```python
from build123d import *

# Parameters (mm, degrees)
F0_W     = 146.05
F0_H     = 41.91
F0_W_2   = 144.78
F0_H_2   = 40.64
F1_DEPTH = 184.15
F2_R     = 12.7
F3_DEPTH = 0.635
F4_W     = 25.654
F4_H     = 44.958
F4_W_2   = 14.224
F4_H_2   = 13.208
F4_R     = 10.16
F4_R_2   = 6.35
F4_R_3   = 2.54
F5_DEPTH = 0.635
F4_R_4   = 1.4859
F6_DEPTH = 0.635


with BuildPart() as f1:
    # F0 (on Front) → F1 (new body)
    with BuildSketch(Plane.XZ):
        with Locations((73.025, 20.955)):
            Rectangle(F0_W, F0_H)
        with Locations((73.025, 20.955)):
            Rectangle(F0_W_2, F0_H_2, mode=Mode.SUBTRACT)
    extrude(amount=-F1_DEPTH)

    # F2 (on face) → F3 (cut, through all)
    with BuildSketch(Plane(origin=(0, 0, 0), x_dir=(1, 0, 0), z_dir=(0, 0, -1))):
        with Locations((19.05, -165.1)):
            Circle(F2_R)
    extrude(amount=-F3_DEPTH, mode=Mode.SUBTRACT)

    # F4 (on face) → F5 (cut, through all)
    with BuildSketch(Plane.XY.offset(41.91)):
        with Locations((25.4, 48.9712)):
            Rectangle(F4_W, F4_H)
        with Locations((25.4, 103.4542)):
            Rectangle(F4_W_2, F4_H_2)
        with Locations((25.4, 148.59)):
            Circle(F4_R)
        with Locations((63.5, 92.075)):
            Circle(F4_R_2)
        with Locations((63.5, 57.785)):
            Circle(F4_R_3)
        with Locations((120.65, 71.755)):
            Circle(F4_R_3)
        with Locations((120.65, 132.715)):
            Circle(F4_R_3)
    extrude(amount=-F5_DEPTH, mode=Mode.SUBTRACT)

    # F4 (on face) → F6 (cut, through all)
    with BuildSketch(Plane.XY.offset(41.91)):
        with Locations((25.4, 130.5941)):
            Circle(F4_R_4)
        with Locations((63.5, 126.365)):
            Circle(F4_R_3)
        with Locations((120.65, 102.235)):
            Circle(F4_R_3)
        with Locations((120.65, 41.275)):
            Circle(F4_R_3)
    extrude(amount=-F6_DEPTH, mode=Mode.SUBTRACT)


solid = f1.part
```
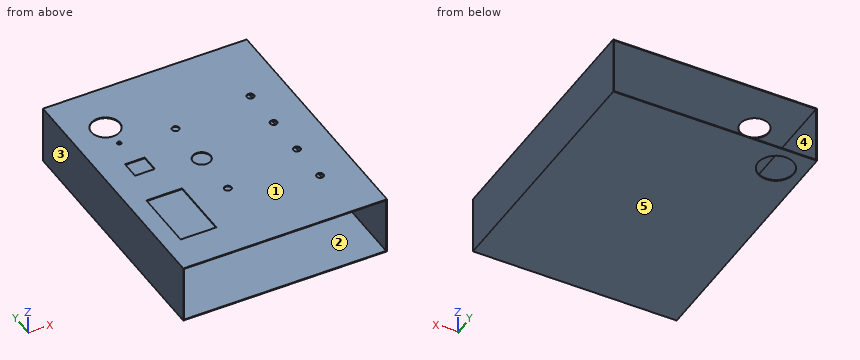
CAD build for the part. Positions are in the model's coordinates, mm. Face numbers are marked on the shaded views. A direction names the side the tool comes from. Round coordinates to 2 decimals unless told otherwise and drop trailing zeros. Order: outer loops, then holes, each group sorted by start corner. A loop starts at its lowest first (then second) coordinate and runs counter-clockwise, first axis right, second up. Notation, with made-up numbers: (43.5, 57.25) -> (62.5, 57.25) arc R26 ccw to (62.5, 79.25) -> close; hole circle Ø9 at (3, -5.5). An arc over 180 degrees is marked (long way). One line per question, with ' | ' between items.
Q1. Slice it at C-C (z = 22.5). Write the cut outline in (x, y) (3 decimals), then the cut area to 3 significant figures.
Completed:
outline: (0, 0) -> (0.635, 0) -> (0.635, 184.15) -> (0, 184.15) -> close; (145.415, 0) -> (146.05, 0) -> (146.05, 184.15) -> (145.415, 184.15) -> close | area: 234 mm^2
Q2. Two-plate mould, pull along Z, no slides. Class the marked faces 3, 4 and 5: released by +Z, released by -Z, zero draft, split by the parting line, or undercut.
Completed:
face 3: zero draft | face 4: undercut | face 5: released by -Z
Q3. Which spindle directions (+Z, -Z, +X, -X, +Y, -Y) get a long thin tool onto all of the face, cutting with end or side? Do the marked faces 1 and 2. Say none if no direction does.
Completed:
face 1: +Z, +X, -X, +Y, -Y | face 2: +Y, -Y
Q4. Slice it at B-B (y = 14). Write the cut outline in (x, z) (3 decimals), then the cut area to 3 significant figures.
Completed:
outline: (0, 0) -> (146.05, 0) -> (146.05, 41.91) -> (0, 41.91) -> close; hole (0.635, 0.635) -> (145.415, 0.635) -> (145.415, 41.275) -> (0.635, 41.275) -> close | area: 237 mm^2
Q5. Probe probe 1 along Y at (x, z) = (120.65, 41.4) (3 decimals); probe 2 along X at (y, z) = (83, 22) (3 decimals); probe 3 along Z at (x, y) = (114, 39.5) (3 decimals). List the from-to ranges inside material, lowest first.
Completed:
probe 1: y = 0 to 38.735, 43.815 to 69.215, 74.295 to 99.695, 104.775 to 130.175, 135.255 to 184.15 | probe 2: x = 0 to 0.635, 145.415 to 146.05 | probe 3: z = 0 to 0.635, 41.275 to 41.91
Q6. Slice it at D-D (y = 148.59). Write the cut outline in (x, z) (3 decimals), then the cut area to 3 significant figures.
Completed:
outline: (0, 0) -> (146.05, 0) -> (146.05, 41.91) -> (35.56, 41.91) -> (35.56, 41.275) -> (145.415, 41.275) -> (145.415, 0.635) -> (0.635, 0.635) -> (0.635, 41.275) -> (15.24, 41.275) -> (15.24, 41.91) -> (0, 41.91) -> close | area: 224 mm^2
Q7. Drop a flat-ended pin along its axis: pin 1 (7.5 mm diameter, centred on x = 63.5, y = 92.075, fed in from +Z) (3 decimals). Give the stop position or say it passes through.
Completed:
pin 1: stops at z = 0.635
Q8. Slice it at A-A (x = 42.5). Write the cut outline in (y, z) (3 decimals), then the cut area to 3 significant figures.
Completed:
outline: (0, 0) -> (184.15, 0) -> (184.15, 0.635) -> (0, 0.635) -> close; (0, 41.275) -> (184.15, 41.275) -> (184.15, 41.91) -> (0, 41.91) -> close | area: 234 mm^2
